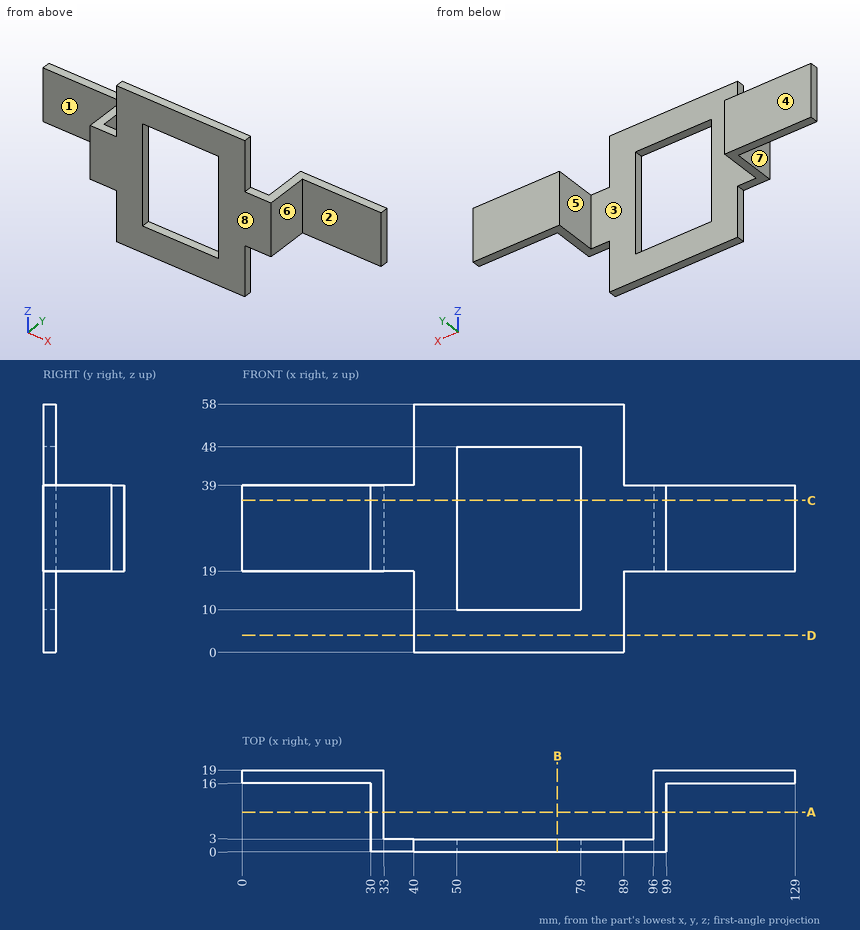
For this review, use the dimensioned drawing (mm, ordinates from the lowest corner) and the shaded views. A direction names the side the tool comes from. Give positions to 0.01 mm unless a question says otherwise; leave off trailing zeros. Write each loop counter-clockwise with the first axis right and the second up, starting at its lowest first coordinate (ties: lowest second). Pieces come first, ordered by that corner, then holes. Notation, with made-up numbers: M 24.25,41.25 L 42.25,41.25 A14 cw 42.25,66.25 Z; hole C -27,77 d2. An arc over 180 degrees is marked long. Answer as a JSON object with one key per item and string values. Group by question number.
Item 1: Draft analysis for pull direction X (two halves, no side actions). For the marked faces 5, 6, 7 and 8, state which applies: +X half, -X half, draft (parallel to the pull), parting line (faces both ways), or undercut.
Item 2: For probe 1 along X at (y, z) = (4.25, 33.5); probe 2 along X at (y, z) = (1, 27.5); probe 3 along Y at (x, z) = (17.5, 26), list the stretches that pass through material, from the lowest coordinate up. Write a range as [from, to].
Item 3: Tool access review of the marked faces 1, 2, 3 and 4: name each direction out of +Z, -Z, +X, -X, +Y, -Y from which nothing blocks a thin tool from reaching the whole face with its end or side.
Item 4: Consider section D-D on z = 4. Write out the cut boundary in (x, y), plus the area to 3 significant figures.
Item 5: Consider section B-B on x = 73.5. Write out the cut boundary in (y, z), plus the area to 3 significant figures.
Item 6: For pin 1 Ø1.5 at (x, y) = (35, 10) entering from -Z; pin 2 Ø6 at (x, z) = (42, 32.5) entering from +Y; pin 3 Ø3.5 at (y, z) = (1, 9.5) entering from -X; pin 4 Ø10 at (x, z) = (13.5, 25.5) entering from -Y, all flat-tipped, find the tip position at first contact; note any pin that passes through.
Item 7: Consider section C-C on z = 35.5. Write out the cut boundary in (x, y).
Item 8: Consider section A-A on y = 9.25. Write out the cut boundary in (x, z), plus the area to 3 significant figures.
Check result:
{
 "1": {"face 5": "undercut", "face 6": "+X half", "face 7": "-X half", "face 8": "draft"},
 "2": {"probe 1": "x = [30, 33], [96, 99]", "probe 2": "x = [30, 50], [79, 99]", "probe 3": "y = [16, 19]"},
 "3": {"face 1": "+Z, -Z, -X, -Y", "face 2": "+Z, -Z, +X, -Y", "face 3": "+Z, -Z, +Y", "face 4": "+Z, -Z, +X, -X, +Y"},
 "4": {"outline": "M 40,0 L 89,0 L 89,3 L 40,3 Z", "area": "147 mm^2"},
 "5": {"outline": "M 0,0 L 3,0 L 3,10 L 0,10 Z; M 0,48 L 3,48 L 3,58 L 0,58 Z", "area": "60.0 mm^2"},
 "6": {"pin 1": "passes through", "pin 2": "stops at y = 3", "pin 3": "stops at x = 40", "pin 4": "stops at y = 16"},
 "7": {"outline": "M 0,16 L 30,16 L 30,0 L 50,0 L 50,3 L 33,3 L 33,19 L 0,19 Z; M 79,0 L 99,0 L 99,16 L 129,16 L 129,19 L 96,19 L 96,3 L 79,3 Z"},
 "8": {"outline": "M 30,19 L 33,19 L 33,39 L 30,39 Z; M 96,19 L 99,19 L 99,39 L 96,39 Z", "area": "120 mm^2"}
}
